Autodesk Inventor part; units mm, degrees
ref_plane "YZ Plane" through (0, 0, 0) normal (1, 0, 0) x (0, 1, 0)
ref_plane "XZ Plane" through (0, 0, 0) normal (0, 1, 0) x (-1, 0, 0)
ref_plane "XY Plane" through (0, 0, 0) normal (0, 0, 1) x (1, 0, 0)
sketch "Sketch1" plane through (0, 0, 0) normal (1, 0, 0) x (0, 1, 0)
  circle A0 centre (28.5689, 30.7216) radius 0.9679
  circle A1 centre (28.5689, -0.2784) radius 0.9679
  circle A2 centre (-2.4311, 30.7216) radius 0.9679
  circle A3 centre (-2.4311, -0.2784) radius 0.9679
  line L0 (-3.9311, 36.2216) -> (30.0689, 36.2216)
  line L1 (34.0689, 32.2216) -> (34.0689, -1.7784)
  line L2 (30.0689, -5.7784) -> (-3.9311, -5.7784)
  line L3 (-7.9311, -1.7784) -> (-7.9311, 32.2216)
  line L4 (-3.9311, 36.2216) -> (-7.9311, 32.2216)
  line L5 (-7.9311, -1.7784) -> (-3.9311, -5.7784)
  line L6 (30.0689, -5.7784) -> (34.0689, -1.7784)
  line L7 (34.0689, 32.2216) -> (30.0689, 36.2216)
  point P0 (-7.9311, 36.2216)
  point P1 (34.0689, -5.7784)
  point P2 (34.0689, 36.2216)
  point P3 (-7.9311, -5.7784)
  dimension "d5" = 31
  dimension "d6" = 31
  dimension "d8" = 31
  dimension "d16" = 42
  dimension "d17" = 42
  dimension "d18" = 5.5
  dimension "d19" = 5.5
  dimension "d21" = 4
  dimension "d22" = 4
  dimension "d23" = 4
  dimension "d24" = 4
  dimension "d25" = 4
  dimension "d26" = 4
  dimension "d27" = 4
  dimension "d28" = 4
extrude "Extrusion1" add sketch "Sketch1" along normal blind 33
sketch "Sketch2" plane through (33, 0, 0) normal (1, 0, 0) x (0, 0, -1)
  circle A0 centre (0.2784, -2.4311) radius 0.9679
  circle A1 centre (-30.7216, -2.4311) radius 0.9679
  circle A2 centre (0.2784, 28.5689) radius 0.9679
  circle A3 centre (-30.7216, 28.5689) radius 0.9679
  line L0 (-36.2216, -3.9311) -> (-32.2216, -7.9311)
  line L1 (-32.2216, -7.9311) -> (1.7784, -7.9311)
  line L2 (1.7784, -7.9311) -> (5.7784, -3.9311)
  line L3 (5.7784, -3.9311) -> (5.7784, 30.0689)
  line L4 (5.7784, 30.0689) -> (1.7784, 34.0689)
  line L5 (1.7784, 34.0689) -> (-32.2216, 34.0689)
  line L6 (-32.2216, 34.0689) -> (-36.2216, 30.0689)
  line L7 (-36.2216, 30.0689) -> (-36.2216, -3.9311)
  circle A4 centre (-15.2216, 13.0689) radius 2.5
  point P0 (0, 0)
  dimension "d29" = 5
extrude "Extrusion2" add sketch "Sketch2" along normal blind 22.3 contours A4
sketch "Sketch3" plane through (33, 0, 0) normal (1, 0, 0) x (0, 0, -1)
  circle A0 centre (-15.2216, 13.0689) radius 2.5
  circle A1 centre (-15.2216, 13.0689) radius 11
  point P0 (0, 0)
  dimension "d32" = 22
extrude "Extrusion3" add sketch "Sketch3" along normal blind 2
properties part number "motor mount"
Design review of the part built by this model. Coordinates are the model's own, in mm. A direction names the side the tool comes from. Give positions to 0.01 mm unless a question says otherwise; leave off trailing zeros. Order: outer loops, then holes, each group sorted by start corner. A loop starts at its lowest first (then second) coordinate and runs counter-clockwise, first axis right, second up. Notation, with made-up numbers: (2, 41.25) -> (44, 41.25) arc R33 cw to (44, 69.25) -> close; hole circle Ø1 at (82.5, 17.5). An arc over 180 degrees is marked (long way). Write each question's results on one line, items separated by ' | '. Start each with the question number.
Q1. Mouldability with a two-part tool opening along Z and no side actions: class faces 3 (the cylindrical face through (16.269, -2.641, 31.666)), 4 (the flat face through (16, 34.069, 15)), 5 (the flat face through (16, 13, -5.778)), 6 (the cylindrical face through (16.269, 29.089, -1.095)) as +Z half, -Z half, draft (parallel to the pull), parting line (faces both ways), or undercut.
Q2. Wall thickness on L1, parallel to Y at x = 29, z = 0; L2, parallel to X at y = 15.5, z = 18.5; L3, parallel to X at y = -4, z = 0.5: over which ranges is each line inside the solid? List them lowest first. Write a range as from..to.
Q3. Add section D-D on x = 39. Give the boundary of the cut face in (y, z), and give its area (3 significant figures).
Q4. Add section B-B on y = 23. Give the boundary of the cut face in (x, z), and give its area (3 significant figures).
Q5. Add section A-A on x = 10. Give the boundary of the cut face in (y, z), and give its area (3 significant figures).
Q6. Add section C-C on z = 11. Give the boundary of the cut face in (x, y).
Q7. For pin 1 (1 mm diameter, centred on y = 20.5, z = 13, fed in from +X); pin 2 (3 mm diameter, centred on x = 36, y = 22.5, fed in from +Z), all flat-tipped, find the tip position at first contact; note any pin that passes through.
Q8. Machinability: for faces 1 (the cylindrical face through (45.01, 12.96, 17.72)), 2 (the cylindrical face through (16.3, -3.4, -0.3)), which of the approach directions +Z, -Z, +X, -X, +Y, -Y give a long, thin tool a straight path to every point of the face, cutting with its end or side? Answer none if there is none.
Found:
1) face 3: undercut | face 4: draft | face 5: -Z half | face 6: undercut
2) L1: y = -7.93..-3.36, -1.5..27.64, 29.5..34.07 | L2: x = 0..35 | L3: x = 0..33
3) outline: circle Ø5 at (13.07, 15.22) | area: 19.6 mm2
4) outline: (0, -5.78) -> (33, -5.78) -> (33, 10.49) -> (35, 10.49) -> (35, 19.95) -> (33, 19.95) -> (33, 36.22) -> (0, 36.22) -> close | area: 1,400 mm2
5) outline: (-7.93, -1.78) -> (-3.93, -5.78) -> (30.07, -5.78) -> (34.07, -1.78) -> (34.07, 32.22) -> (30.07, 36.22) -> (-3.93, 36.22) -> (-7.93, 32.22) -> close; hole circle Ø1.94 at (-2.43, -0.28); hole circle Ø1.94 at (-2.43, 30.72); hole circle Ø1.94 at (28.57, -0.28); hole circle Ø1.94 at (28.57, 30.72) | area: 1,720 mm2
6) outline: (0, -7.93) -> (33, -7.93) -> (33, 2.91) -> (35, 2.91) -> (35, 23.23) -> (33, 23.23) -> (33, 34.07) -> (0, 34.07) -> close
7) pin 1: stops at x = 35 | pin 2: stops at z = 22.43
8) face 1: +X | face 2: +X, -X
